Check sheet for the modelled part. Datum: model origin and axes. Units: mm. A direction names the side the tool comes from. Coordinates: 2 decimals unless noted, no trailing zeros. Write each loop counter-clockwise with the first axis right and the second up, starting at its lowest first coordinate (ties: lowest second). Pieces come first, ordered by that corner, then holes. Notation, with made-up numbers: M -15.75,58 L 20.25,58 A10 ccw 20.25,72 Z; hole C 71.5,-13.75 d1. An arc over 180 degrees is marked long. Answer as CSV lines item,"result".
from build123d import *

# Parameters (mm, degrees)
F1_DEPTH       = 50.8
F3_D           = 7.874
F3_CBORE_D     = 12.7
F3_CBORE_DEPTH = 6.096
F6_DEPTH       = 134.531275
F8_DEPTH       = 54.103


with BuildPart() as f1:
    # F0 (on Front) → F1 (new body)
    with BuildSketch(Plane.XZ):
        Polygon((0, 12.7), (0, 0), (85.852, 0), (131.70327, -45.85127), (149.663782, -27.890758), (111.587496, 10.185528), (102.60724, 1.205272), (91.112512, 12.7), align=None)
    extrude(amount=F1_DEPTH)

    # F3 (through all)
    with Locations(Plane(origin=(0, 0, 0), x_dir=(1, 0, 0), z_dir=(0, 0, -1))):
        with Locations((15.748, 38.1), (69.596, 38.1), (69.596, 12.7), (15.748, 12.7)):
            CounterBoreHole(F3_D / 2, F3_CBORE_D / 2, F3_CBORE_DEPTH)

    # F5 (on face) → F6 (cut, through all)
    with BuildSketch(Plane(origin=(88.77727, 0, -88.77727), x_dir=(0, 1, 0), z_dir=(0.707107, 0, -0.707107))):
        Polygon((-15.748, 86.106531), (-35.052, 86.106531), (-35.052, 80.010531), (-41.148, 80.010531), (-41.148, 73.914531), (-9.652, 73.914531), (-9.652, 80.010531), (-15.748, 80.010531), align=None)
    extrude(amount=-F6_DEPTH, mode=Mode.SUBTRACT)

    # F7 (on face) → F8 (cut, through all)
    with BuildSketch(Plane(origin=(42.926, 0, 42.926), x_dir=(0.707107, 0, -0.707107), z_dir=(-0.707107, 0, -0.707107))):
        with BuildLine():
            ThreePointArc((119.183037, 50.8), (123.934026, 38.492922), (125.550019, 25.4))
            Line((125.550019, 25.4), (125.550019, 50.8))
            Line((125.550019, 50.8), (119.183037, 50.8))
        make_face()
        with BuildLine():
            ThreePointArc((125.550019, 25.4), (123.934026, 12.307078), (119.183037, 0))
            Line((119.183037, 0), (125.550019, 0))
            Line((125.550019, 0), (125.550019, 25.4))
        make_face()
    extrude(amount=-F8_DEPTH, mode=Mode.SUBTRACT)


solid = f1.part
1) Mould release check, pull along Y, two halves, no side actions. Record for faces 1 (the face through (73.01, -18.054, 3.005)), 2 (the face through (88.4, 0, -2.2)), 3 (the face through (74, -38, 6.096)), 4 (the face through (0, -25, 6)): pulls with the +Y half, pulls with the -Y half, needs draft (parallel to the pull), parting line crosses it, or undercut.
Answer key:
face 1,"undercut"
face 2,"pulls with the +Y half"
face 3,"undercut"
face 4,"needs draft"
2) Depth check by flat-ended pin: P1, Ø11.5, axis at x = 69.596, y = -12.7, coming from the -Z side; P2, Ø4.5, axis at x = 69.596, y = -38.1, coming from the -Z side; P3, Ø2, axis at x = 94.5, y = -13.5, coming from the -Z side; P4, Ø5, axis at y = -39, z = -3, coming from the +X side. Enter the tip coordinate at first touch or a pass-through.
Answer key:
P1,"stops at z = 6.1"
P2,"passes through"
P3,"stops at z = -9.65"
P4,"stops at x = 127.27"
3) Thickness scan on line 1 along X through (y, z) = (-37, 6); line 2 along Z through (x, y) = (33.5, -5); line 3 along X through (y, z) = (-38, 11). Record the ranges inside material, lowest first.
Answer key:
line 1,"x = 0 to 9.49, 22 to 63.34, 75.85 to 97.81, 107.4 to 115.77"
line 2,"z = 0 to 12.7"
line 3,"x = 0 to 11.81, 19.68 to 65.66, 73.53 to 92.81"
4) Section check C-C, the plane x = 15.5. Record the boundary of the cut face in (y, z).
Answer key:
outline,"M -50.8,0 L -44.45,0 L -44.45,6.1 L -42.03,6.1 L -42.03,12.7 L -50.8,12.7 Z; M -34.17,6.1 L -31.75,6.1 L -31.75,0 L -19.05,0 L -19.05,6.1 L -16.63,6.1 L -16.63,12.7 L -34.17,12.7 Z; M -8.77,6.1 L -6.35,6.1 L -6.35,0 L 0,0 L 0,12.7 L -8.77,12.7 Z"
5) Section check A-A, the plane z = 3. Record the boundary of the cut face in (x, y), plus the area to 3 significant figures.
Answer key:
outline,"M 0,-50.8 L 100.81,-50.8 L 100.81,0 L 0,0 Z; M 104.4,-50.8 L 118.77,-50.8 L 118.77,-35.05 L 110.15,-35.05 L 110.15,-41.15 L 104.4,-41.15 Z; M 104.4,-9.65 L 110.15,-9.65 L 110.15,-15.75 L 118.77,-15.75 L 118.77,0 L 104.4,0 Z; hole C 15.75,-38.1 d12.7; hole C 15.75,-12.7 d12.7; hole C 69.6,-38.1 d12.7; hole C 69.6,-12.7 d12.7"
area,"5,000 mm2"
6) Section check D-D, the plane z = -13.5. Record the boundary of the cut face in (x, y).
Answer key:
outline,"M 99.35,-50.8 L 135.27,-50.8 L 135.27,-35.05 L 126.65,-35.05 L 126.65,-41.15 L 118.03,-41.15 L 118.03,-9.65 L 126.65,-9.65 L 126.65,-15.75 L 135.27,-15.75 L 135.27,0 L 99.35,0 Z"
7) Tool access check on faces 5 (the face through (126.27, -38.06, -13.12)), 6 (the face through (128, -35.052, -11)), 7 (the face through (19.162, -18.054, 3.005)), 8 (the face through (96.94, -25.04, 6.87)). Record the directions out of +Z, -Z, +X, -X, +Y, -Y that give a thin tool (end or side, any length) a straight path to the whole face; none if there is none.
Answer key:
face 5,"none"
face 6,"+Z, +X"
face 7,"-Z"
face 8,"+Z, +Y, -Y"
8) Section check B-B, the plane y = -12.7. Record the boundary of the cut face in (x, z) (1 decimal).
Answer key:
outline,"M 0,0 L 9.4,0 L 9.4,6.1 L 11.8,6.1 L 11.8,12.7 L 0,12.7 Z; M 19.7,6.1 L 22.1,6.1 L 22.1,0 L 63.2,0 L 63.2,6.1 L 65.7,6.1 L 65.7,12.7 L 19.7,12.7 Z; M 73.5,6.1 L 75.9,6.1 L 75.9,0 L 85.9,0 L 130.6,-44.8 L 140,-35.4 L 103,1.6 L 102.6,1.2 L 91.1,12.7 L 73.5,12.7 Z; M 107.3,5.9 L 144.3,-31.1 L 148.6,-26.8 L 111.6,10.2 Z"
